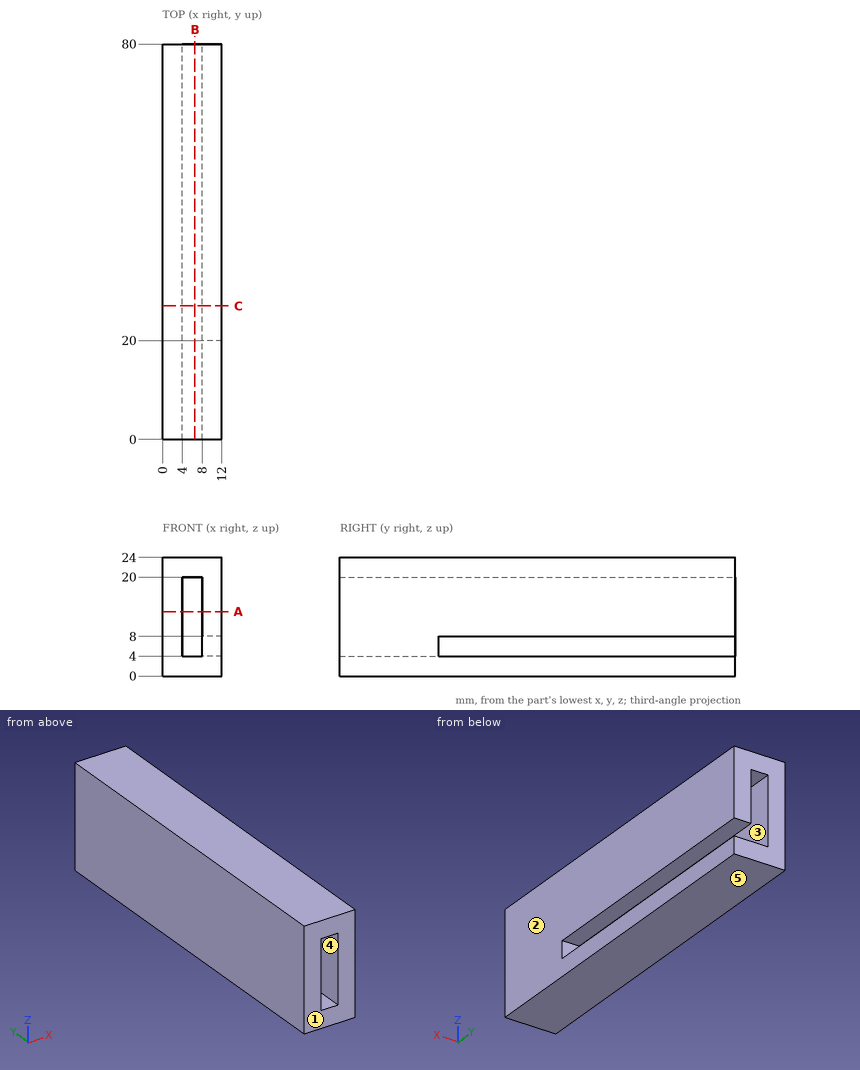
Here's the drawing with two shaded views (mm, measured from the low corner). I have some questions. A direction names the side the tool comes from. Round coordinates to 2 decimals unless told otherwise and drop trailing zeros. Loops run counter-clockwise (first coordinate to the right, second up) from the corner with the lowest first, then second, coordinate; pieces in that order, holes last. Notation, with made-up numbers: M 10.25,36.5 L 26.25,36.5 A34 ccw 26.25,70.5 Z; hole C 65.25,3 d8. An arc over 180 degrees is marked long. Answer as a JSON object with one key per item and string values. Group by question number.
Q1. Imagine slicing it at C-C, the plane y = 27. Please give me the cut outline in (x, z).
Q2. Imagine slicing it at A-A, the plane z = 13. Please give me the cut outline in (x, y).
Q3. Imagine slicing it at B-B, the plane x = 6.5. Please give me the cut outline in (y, z).
Q4. On a 3-axis mill with a long thin cutter (end or side, diameter ignored), from which of +Z, -Z, +X, -X, +Y, -Y can I reach the whole of each face in a straight line? I mean the marked faces 4 and 5. Say none if no direction works.
Q5. Please list where these lines run through material, in increasing order: L1, parallel to Z at x = 9.5, y = 53.5; L2, parallel to X at y = 50, z = 11.5; L3, parallel to Z at x = 6, y = 28.
Q6. Will this pin go through, and if not, where does the flat tip stop? pin 1 (1.2 mm diameter, centred on x = 10, y = 49, fed in from -Z).
Q7. We'd pull the mould along X, two halves only. Please class the marked faces 1, 2 and 3: +X half, -X half, draft (parallel to the pull), parting line (faces both ways), or undercut.
Findings:
{
 "1": {"outline": "M 0,0 L 12,0 L 12,4 L 4,4 L 4,20 L 8,20 L 8,8 L 12,8 L 12,24 L 0,24 Z"},
 "2": {"outline": "M 0,0 L 4,0 L 4,80 L 0,80 Z; M 8,0 L 12,0 L 12,80 L 8,80 Z"},
 "3": {"outline": "M 0,0 L 80,0 L 80,4 L 0,4 Z; M 0,20 L 80,20 L 80,24 L 0,24 Z"},
 "4": {"face 4": "+Y, -Y", "face 5": "-Z, +X, -X, +Y, -Y"},
 "5": {"L1": "z = 0 to 4, 8 to 24", "L2": "x = 0 to 4, 8 to 12", "L3": "z = 0 to 4, 20 to 24"},
 "6": {"pin 1": "stops at z = 0"},
 "7": {"face 1": "draft", "face 2": "+X half", "face 3": "undercut"}
}
